from build123d import *

# Parameters (mm, degrees)
SKETCH1_W                = 17.78
SKETCH1_H                = 4.064
BOSS_EXTRUDE1_DEPTH      = 6.35
FILLET1_RADIUS           = 2.032
FILLET1_LENGTH           = 17.78
SKETCH2_R                = 1.532
BOSS_EXTRUDE2_DEPTH      = 2
CHAMFER1_SIZE            = 0.3
CHAMFER1_OF_MIRROR1_SIZE = 0.3
SKETCH3_W                = 6.096
SKETCH3_H                = 3.048
BOSS_EXTRUDE3_DEPTH      = 4.7625
SKETCH4_W                = 6.096
SKETCH4_H                = 4.7625
BOSS_EXTRUDE4_DEPTH      = 0.127
CHAMFER2_SIZE            = 1


with BuildPart() as part:
    # Sketch1 → Boss-Extrude1 (new body)
    with BuildSketch(Plane.XY):
        with Locations((-3503.971479642, 500.3673)):
            Rectangle(SKETCH1_W, SKETCH1_H)
    extrude(amount=BOSS_EXTRUDE1_DEPTH)

    # Fillet1: full round fillet: the end face becomes a half cylinder, R = half its width
    fillet1_face = Plane((-3503.971479642, 500.3673, 6.35), x_dir=(1, 0, 0), z_dir=(0, 0, 1))  # on the end face: x along it, z out of the body
    fillet1_slab = fillet1_face.offset(-FILLET1_RADIUS / 2) * Box(FILLET1_LENGTH, 2 * FILLET1_RADIUS, FILLET1_RADIUS, mode=Mode.PRIVATE)  # the body's end, R deep
    fillet1_round = Plane((-3503.971479642, 500.3673, 4.318), x_dir=(0, 0, 1), z_dir=(1, 0, 0)) * Cylinder(FILLET1_RADIUS, FILLET1_LENGTH, mode=Mode.PRIVATE)  # its axis R under the face
    add(fillet1_slab - fillet1_round, mode=Mode.SUBTRACT)

    # Sketch2 → Boss-Extrude2 (add)
    with BuildSketch(Plane.ZY.offset(3512.861479642)):
        with Locations(Location((4.318, 500.3673, 0), (0, 0, 180))):
            Circle(SKETCH2_R)
    boss_extrude2 = extrude(amount=BOSS_EXTRUDE2_DEPTH)

    # Chamfer1
    chamfer1_edges = [part.edges().sort_by_distance(p)[0] for p in [
        (-3514.861479642, 500.3673, 5.85),
    ]]
    chamfer(chamfer1_edges, length=CHAMFER1_SIZE)

    # Mirror1: Boss-Extrude2 across plane
    add(boss_extrude2.mirror(Plane.ZY.offset(3503.971479642)))

    # Chamfer1 of Mirror1
    chamfer1_of_mirror1_edges = [part.edges().sort_by_distance(p)[0] for p in [
        (-3493.081479642, 500.3673, 5.85),
    ]]
    chamfer(chamfer1_of_mirror1_edges, length=CHAMFER1_OF_MIRROR1_SIZE)

    # Sketch3 → Boss-Extrude3 (add)
    with BuildSketch(Plane(origin=(0, 0, 0), x_dir=(-1, 0, 0), z_dir=(0, 0, -1))):
        with Locations((3503.971479642, 499.9863)):
            Rectangle(SKETCH3_W, SKETCH3_H)
    extrude(amount=BOSS_EXTRUDE3_DEPTH)

    # Sketch4 → Boss-Extrude4 (add)
    with BuildSketch(Plane.XZ.offset(-498.4623)):
        with Locations((-3503.971479642, -2.38125)):
            Rectangle(SKETCH4_W, SKETCH4_H)
    extrude(amount=BOSS_EXTRUDE4_DEPTH)

    # Chamfer2
    chamfer2_edges = [part.edges().sort_by_distance(p)[0] for p in [
        (-3500.923479642, 499.9228, -4.7625),
        (-3507.019479642, 499.9228, -4.7625),
    ]]
    chamfer(chamfer2_edges, length=CHAMFER2_SIZE)


solid = part.part
The model under review builds one solid part; all positions refer to its coordinate system, in mm. A direction names the side the tool comes from. Round coordinates to 2 decimals unless told otherwise and drop trailing zeros. Loops run counter-clockwise (first coordinate to the right, second up) from the corner with the lowest first, then second, coordinate; pieces in that order, holes last. Notation, with made-up numbers: M -35.5,42.25 L -25.5,42.25 A22 cw -25.5,53.25 Z; hole C -2,-29.5 d11. An arc over 180 degrees is marked long. Answer as a JSON object with one key per item and string values.
Item 1: We need section B-B, the plane z = 2. State the section outline as (x, y) points.
Check sheet entries:
{"outline": "M -3512.86,498.34 L -3495.08,498.34 L -3495.08,502.4 L -3512.86,502.4 Z"}
Item 2: Tool access review of faces 1 (the face through (-3500.923, 500, -2)), 2 (the face through (-3507.019, 500, -2)), 3 (the face through (-3494.243, 501.863, 4.65)), 4 (the face through (-3513.7, 501.863, 4.65)): name each direction out of +Z, -Z, +X, -X, +Y, -Y from which nothing blocks a thin tool from reaching the whole face with its end or side.
Check sheet entries:
{"face 1": "-Z, +X, +Y, -Y", "face 2": "-Z, -X, +Y, -Y", "face 3": "+X", "face 4": "-X"}
Item 3: We need section C-C, the plane z = -0.5. State the section outline as (x, y) points, and give its area (3 significant figures).
Check sheet entries:
{"outline": "M -3507.02,498.34 L -3500.92,498.34 L -3500.92,501.51 L -3507.02,501.51 Z", "area": "19.4 mm2"}
Item 4: We need section A-A, the plane x = -3502.5. State the section outline as (y, z) points, and give its area (3 significant figures).
Check sheet entries:
{"outline": "M 498.34,-4.76 L 501.51,-4.76 L 501.51,0 L 502.4,0 L 502.4,4.32 A2.03 ccw 498.34,4.32 Z", "area": "39.2 mm2"}
Item 5: For line 1 along X through (y, z) = (499.55, -3.25); line 2 along X through (y, z) = (498.7, 0.25); line 3 along Z through (x, y) = (-3512.5, 500.25), list the stretches that pass through material, from the lowest coordinate up.
Check sheet entries:
{"line 1": "-3507.02 to -3500.92", "line 2": "-3512.86 to -3495.08", "line 3": "0 to 6.35"}
Item 6: Clearance check with flat-ended pins moving along their axes: P1, Ø1.5, axis at y = 501, z = -3.5, coming from the -X side; P2, Ø1.5, axis at x = -3510, z = -2.5, coming from the +Y side; P3, Ø1, axis at y = 499.5, z = -2.5, coming from the +X side; P4, Ø2.5, axis at x = -3504.5, z = -3.5, coming from the +Y side. State where each tip first meets the part, or that it passes through.
Check sheet entries:
{"P1": "x = -3507.02", "P2": "through", "P3": "x = -3500.92", "P4": "y = 501.51"}
